Verification items for the finished model (mm, model axes). A direction names the side the tool comes from. Coordinates: 2 decimals unless noted, no trailing zeros. Order: outer loops, then holes, each group sorted by start corner. A loop starts at its lowest first (then second) coordinate and runs counter-clockwise, first axis right, second up. Notation, with made-up numbers: (-29.5, 4.5) -> (16.5, 4.5) arc R27 ccw to (16.5, 34.5) -> close; hole circle Ø2 at (54.25, 6). An arc over 180 degrees is marked (long way). Write item = value, one per line. Start each with the question number.
1. Cross-section at D-D on z = 27.5. Record the cut outline in (x, y), plus the area to 3 significant figures.
2. Thickness scan on line 1 along Y through (x, z) = (49.5, 30); line 2 along X through (y, z) = (-0.35, -6); line 3 along Z through (x, y) = (-38, -0.75). Record the ranges inside material, lowest first. Write a range as from..to.
3. Cross-section at A-A on z = 0. Record the cut outline in (x, y) (3 decimals), plus the area to 3 significant figures.
4. Cross-section at B-B on x = 0. Record the cut outline in (y, z) (3 decimals).
5. Cross-section at C-C on y = 1.15. Record the cut outline in (x, z).
6. Go/stop test with flat-tipped pins: P1, Ø6, axis at x = -21.5, z = -31, coming from the +Y side; P2, Ø3, axis at y = 0.5, z = 27.5, coming from the +X side; P3, Ø1, axis at y = 1.5, z = -37, coming from the +X side; P4, Ø3, axis at x = -13.5, z = -7, coming from the -Y side. Record where each tip stops, or that it passes through.
7. Release check for a two-part mould opening along Y. For faces 1 (the flat face through (-1, 0, -13)), 2 (the cylindrical face through (0.867, 1.109, -3.905)), 3 (the flat face through (0, -3, 0)) record: +Y half, -Y half, draft (parallel to the pull), parting line (faces both ways), or undercut.
8. Set-up check for faces 4 (the cylindrical face through (-0.867, -1.986, -3.905)), 5 (the cylindrical face through (-60.267, -0.493, 2.652)): record each of +Z, -Z, +X, -X, +Y, -Y from which the full face is reachable in a straight line by a thin tool's end or side.
from build123d import *

# Parameters (mm, degrees)
F1_R     = 4
F2_DEPTH = 3
F0_R     = 60.325
F3_DEPTH = 1
F4_R     = 4
F5_DEPTH = 2.25


with BuildPart() as f2:
    # F1 (on face) → F2 (new body)
    with BuildSketch(Plane.XZ):
        Circle(F1_R)
    extrude(amount=F2_DEPTH)

    # F0 (on Front) → F3 (join)
    with BuildSketch(Plane.XZ):
        Circle(F0_R)
    extrude(amount=F3_DEPTH)

    # F4 (on face) → F5 (join)
    with BuildSketch(Plane(origin=(0, 0, 0), x_dir=(-1, 0, 0), z_dir=(0, 1, 0))):
        Circle(F4_R)
    extrude(amount=F5_DEPTH)


solid = f2.part
Worked out:
q1.outline = (-53.69, -1) -> (53.69, -1) -> (53.69, 0) -> (-53.69, 0) -> close
q1.area = 107 mm²
q2.line_1 = -1..0
q2.line_2 = -60.03..60.03
q2.line_3 = -46.85..46.85
q3.outline = (-60.325, -1) -> (-4, -1) -> (-4, -3) -> (4, -3) -> (4, -1) -> (60.325, -1) -> (60.325, 0) -> (4, 0) -> (4, 2.25) -> (-4, 2.25) -> (-4, 0) -> (-60.325, 0) -> close
q3.area = 155 mm²
q4.outline = (-3, -4) -> (-1, -4) -> (-1, -60.325) -> (0, -60.325) -> (0, -4) -> (2.25, -4) -> (2.25, 4) -> (0, 4) -> (0, 60.325) -> (-1, 60.325) -> (-1, 4) -> (-3, 4) -> close
q5.outline = circle Ø8 at (0, 0)
q6.P1 = 0
q6.P2 = 54.39
q6.P3 = through
q6.P4 = -1
q7.face_1 = +Y half
q7.face_2 = draft
q7.face_3 = -Y half
q8.face_4 = -Y
q8.face_5 = +Y, -Y
